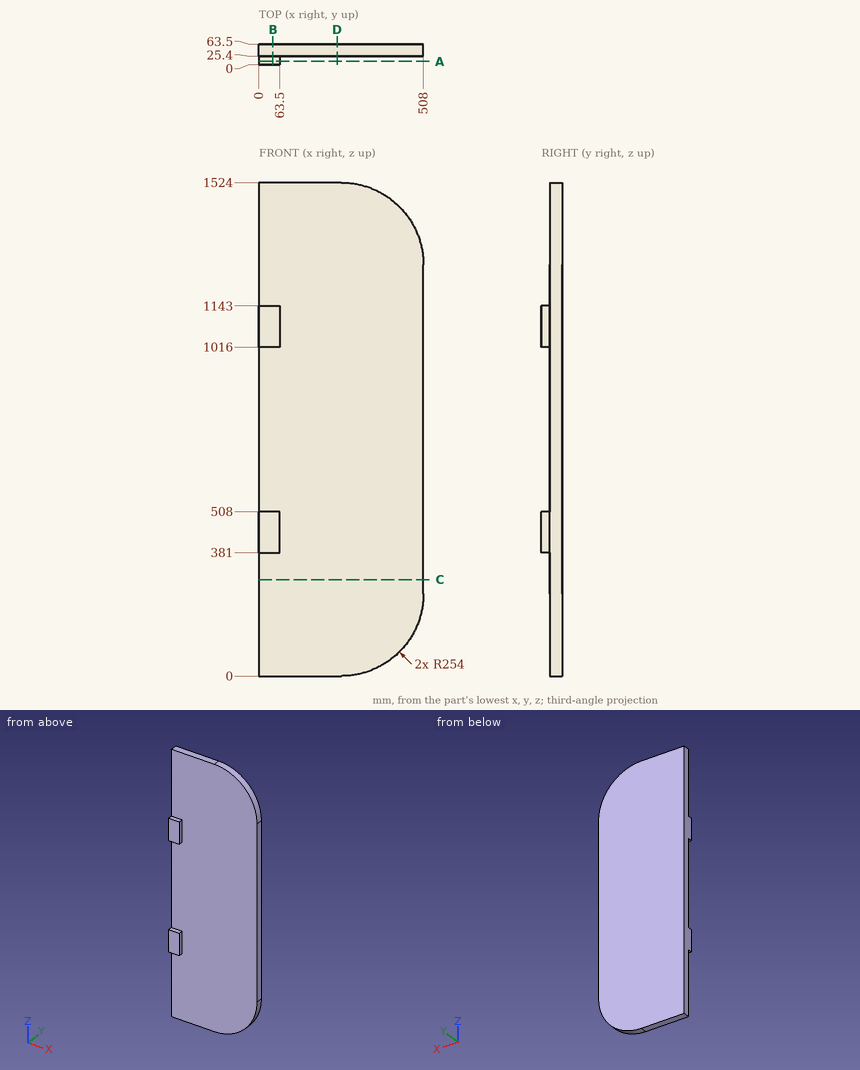
Here's the drawing with two shaded views (mm, measured from the low corner). I have some questions. Give positions to 0.01 mm unless a question says otherwise; leave off trailing zeros. Loops run counter-clockwise (first coordinate to the right, second up) from the corner with the lowest first, then second, coordinate; pieces in that order, holes last. Notation, with made-up numbers: M -33,-27.5 L -6,-27.5 A29 cw -6,-6.5 Z; hole C -30,57.25 d10. An arc over 180 degrees is marked long. One line per item, written item: value. Start each with the question number.
1) If we section it at C-C, the plane z = 298: Write out the boundary of the cut face in (x, y), and give its area (3 significant figures).
2) I'm going to push flat-ended pins straight in: pin 1 (20.5 mm diameter, centred on x = 36, y = 14.5, fed in from -Z); pin 2 (20.5 mm diameter, centred on x = 34, y = 11.5, fed in from +Z); pin 3 (2 mm diameter, centred on x = 260.5, z = 703.5, fed in from -Y). Where does each tip first touch, or does it pass through?
3) If we section it at A-A, the plane y = 10: Write out the boundary of the cut face in (x, z).
4) If we section it at D-D, the plane x = 241: Write out the boundary of the cut face in (y, z), and give its area (3 significant figures).
5) If we section it at B-B, the plane x = 43: Write out the boundary of the cut face in (y, z), and give its area (3 significant figures).
6) If I drill on line 1 (Y direction, x = 309.5, z = 1104); line 2 (Z direction, x = 374.5, y = 37.5); line 3 (Z direction, x = 484.5, y = 35), over which ranges is the centre line in solid material (lowest first)? Write a range as [from, to].
Completed:
1. outline: M 0,25.4 L 508,25.4 L 508,63.5 L 0,63.5 Z
1. area: 19,400 mm^2
2. pin 1: stops at z = 381
2. pin 2: stops at z = 1143
2. pin 3: stops at y = 25.4
3. outline: M 0,381 L 63.5,381 L 63.5,508 L 0,508 Z; M 0,1016 L 63.5,1016 L 63.5,1143 L 0,1143 Z
4. outline: M 25.4,0 L 63.5,0 L 63.5,1524 L 25.4,1524 Z
4. area: 58,100 mm^2
5. outline: M 0,381 L 25.4,381 L 25.4,0 L 63.5,0 L 63.5,1524 L 25.4,1524 L 25.4,1143 L 0,1143 L 0,1016 L 25.4,1016 L 25.4,508 L 0,508 Z
5. area: 64,500 mm^2
6. line 1: y = [25.4, 63.5]
6. line 2: z = [30.4, 1493.6]
6. line 3: z = [147.3, 1376.7]
